The listing builds one solid part. Answer for the finished solid, in the listing's coordinates (mm). A direction names the side the tool comes from. Round coordinates to 2 decimals unless told otherwise and drop trailing zeros. Write each loop counter-clockwise with the first axis right and the second up, starting at its lowest first coordinate (ties: lowest second). Pieces come first, ordered by that corner, then holes.
(1) A cutting plane is placed at A-A, the plane x = 21. Give the vertices of the cut face in (y, z).
(2) Each of these flat-tipped pins is pushed along its axis until it touches: pin 1 Ø2.5 at (x, y) = (158, 23.5) entering from -Z; pin 2 Ø5 at (y, z) = (28.5, -35) entering from -X; pin 3 Ø4.5 at (x, z) = (4, -31.5) entering from -Y; pin 4 Ø0.9 at (x, z) = (11, -59) entering from -Y. Where does it stop, or does it pass through?
(3) Find the intervals of material crossed by probe 1 along Z at (x, y) = (129, 25); probe 2 along X at (y, z) = (31.75, -39); probe 3 along X at (y, z) = (32.75, -30.5), in increasing order.
(4) For faces 4 (the face through (5, 28.5, -39)), 5 (the face through (191, 30, -39)), 6 (the face through (200, 30, -40)), determine the directions among +Z, -Z, +X, -X, +Y, -Y from which every point of the face is accessible in a straight line to the end or side of a thin tool.
(5) The mould has two halves that part along Z. Classify faces 1 (the face through (9, 30, -39)), 2 (the face through (0, 31, -40)), 3 (the face through (99, 26, -84)): +Z half, -Z half, draft (parallel to the pull), parting line (faces both ways), or undercut.
(6) A cutting plane is placed at B-B, the plane z = -60. Give the vertices of the cut face in (x, y), and give its area (3 significant figures).
from build123d import *

# Parameters (mm, degrees)
SKETCH1_R                 = 1.5
MOUNTING_PLATE_DEPTH      = 4
RAILS_DEPTH               = 80
SKETCH1_4_W               = 91
SKETCH1_4_H               = 5
MOUNTING_PLATE_2_DEPTH    = 4
SKETCH4_W                 = 200
SKETCH4_H                 = 18.5
UNNECESSARY_PLASTIC_DEPTH = 222.057119315


with BuildPart() as part:
    # Sketch1 → Mounting Plate (new body)
    with BuildSketch(Plane.XY):
        Polygon((0, 0), (200, 0), (200, 33.5), (191, 33.5), (191, 28.5), (9, 28.5), (9, 33.5), (0, 33.5), align=None)
        with Locations((158, 23.5)):
            Circle(SKETCH1_R, mode=Mode.SUBTRACT)
        with Locations((42, 23.5)):
            Circle(SKETCH1_R, mode=Mode.SUBTRACT)
    mounting_plate = extrude(amount=MOUNTING_PLATE_DEPTH)

    # Sketch3 → Rails (add)
    with BuildSketch(Plane(origin=(0, 0, 0), x_dir=(-1, 0, 0), z_dir=(0, 0, -1))):
        Polygon((0, 28.5), (0, 33.5), (-12, 33.5), (-12, 32), (-9, 32), (-9, 28.5), align=None)
        Polygon((-188, 32), (-188, 33.5), (-200, 33.5), (-200, 28.5), (-191, 28.5), (-191, 32), align=None)
    extrude(amount=RAILS_DEPTH)

    # Sketch1_4 → Mounting Plate 2 (add)
    with BuildSketch(Plane.XY):
        with Locations((54.5, 31)):
            Rectangle(SKETCH1_4_W, SKETCH1_4_H)
        with Locations((145.5, 31)):
            Rectangle(SKETCH1_4_W, SKETCH1_4_H)
    mounting_plate_2 = extrude(amount=MOUNTING_PLATE_2_DEPTH)

    # Mirror1: Mounting Plate, Mounting Plate 2 across plane
    add(mounting_plate.mirror(Plane.XY.offset(-40)))
    add(mounting_plate_2.mirror(Plane.XY.offset(-40)))

    # Sketch4 → Unnecessary Plastic (cut, through all)
    with BuildSketch(Plane(origin=(0, 0, -84), x_dir=(-1, 0, 0), z_dir=(0, 0, -1))):
        with Locations((-100, 9.25)):
            Rectangle(SKETCH4_W, SKETCH4_H)
    extrude(amount=-UNNECESSARY_PLASTIC_DEPTH, mode=Mode.SUBTRACT)


solid = part.part
Solutions:
1. outline: (18.5, -84) - (33.5, -84) - (33.5, -80) - (18.5, -80) - close; (18.5, 0) - (33.5, 0) - (33.5, 4) - (18.5, 4) - close
2. pin 1: passes through
2. pin 2: stops at x = 0
2. pin 3: stops at y = 28.5
2. pin 4: stops at y = 32
3. probe 1: z = -84 to -80, 0 to 4
3. probe 2: x = 0 to 9, 191 to 200
3. probe 3: x = 0 to 12, 188 to 200
4. face 4: +X, -X, -Y
4. face 5: -Y
4. face 6: +Z, -Z, +X, +Y, -Y
5. face 1: undercut
5. face 2: draft
5. face 3: -Z half
6. outline: (0, 28.5) - (9, 28.5) - (9, 32) - (12, 32) - (12, 33.5) - (0, 33.5) - close; (188, 32) - (191, 32) - (191, 28.5) - (200, 28.5) - (200, 33.5) - (188, 33.5) - close
6. area: 99.0 mm2
